```python
from build123d import *

# Parameters (mm, degrees)
SKETCH2_R               = 27.178
BOSS_EXTRUDE1_DEPTH     = 10
BOSS_EXTRUDE2_START     = -28
BOSS_EXTRUDE2_DEPTH     = 28
SHELL1_START            = -10
SHELL1_DEPTH            = 36
SHELL1_2_DEPTH          = 8
CUT_EXTRUDE3_DEPTH      = 10
CUT_EXTRUDE4_DEPTH      = 47.115916344
CUT_EXTRUDE4_DEPTH_BACK = 47.115916344
SKETCH6_R               = 1.75
SKETCH7_R               = 4
CUT_EXTRUDE6_DEPTH      = 47.115916478


# Read off the part's stored shape, not the designer's step: Shell1
with BuildPart() as part:
    # Sketch2 → Boss-Extrude1 (new body)
    with BuildSketch(Plane(origin=(0, 0, 0), x_dir=(1, 0, 0), z_dir=(0, 1, 0))):
        with Locations(Location((0, 0, 0), (0, 0, 270))):
            Circle(SKETCH2_R)
    extrude(amount=-BOSS_EXTRUDE1_DEPTH)

    # Sketch3 → Boss-Extrude2 (add)
    with BuildSketch(Plane(origin=(0, 0, 0), x_dir=(-1, 0, 0), z_dir=(0, -1, 0)).offset(BOSS_EXTRUDE2_START)):
        with BuildLine():
            Line((-23.587998728, 13.5), (-20.913788663, 13.5))
            ThreePointArc((-20.913788663, 13.5), (-13.609833087, 20.842480649), (-3.95, 24.57710431))
            Line((-3.95, 24.57710431), (-3.95, 20))
            ThreePointArc((-3.95, 20), (0, 16.05), (3.95, 20))
            Line((3.95, 20), (3.95, 24.57710431))
            ThreePointArc((3.95, 24.57710431), (13.609833087, 20.842480649), (20.913788663, 13.5))
            Line((20.913788663, 13.5), (23.587998728, 13.5))
            ThreePointArc((23.587998728, 13.5), (27.178, 0), (23.587998728, -13.5))
            Line((23.587998728, -13.5), (20.913788663, -13.5))
            ThreePointArc((20.913788663, -13.5), (13.609833087, -20.842480649), (3.95, -24.57710431))
            Line((3.95, -24.57710431), (3.95, -20))
            ThreePointArc((3.95, -20), (0, -16.05), (-3.95, -20))
            Line((-3.95, -20), (-3.95, -24.57710431))
            ThreePointArc((-3.95, -24.57710431), (-13.609833087, -20.842480649), (-20.913788663, -13.5))
            Line((-20.913788663, -13.5), (-23.587998728, -13.5))
            ThreePointArc((-23.587998728, -13.5), (-27.178, 0), (-23.587998728, 13.5))
        make_face()
    extrude(amount=BOSS_EXTRUDE2_DEPTH)

    # Shell1 outline → Shell1 (cut)
    with BuildSketch(Plane(origin=(0, 0, 0), x_dir=(1, 0, 0), z_dir=(0, 1, 0)).offset(SHELL1_START)):
        with BuildLine():
            ThreePointArc((22.398251807, -11.5), (25.178, 0), (22.398251807, 11.5))
            Line((22.398251807, 11.5), (19.794356677, 11.5))
            ThreePointArc((19.794356677, 11.5), (13.921689669, 18.172867496), (5.95, 22.105747132))
            Line((5.95, 22.105747132), (5.95, 20))
            ThreePointArc((5.95, 20), (0, 14.05), (-5.95, 20))
            Line((-5.95, 20), (-5.95, 22.105747132))
            ThreePointArc((-5.95, 22.105747132), (-13.921689669, 18.172867496), (-19.794356677, 11.5))
            Line((-19.794356677, 11.5), (-22.398251807, 11.5))
            ThreePointArc((-22.398251807, 11.5), (-25.178, 0), (-22.398251807, -11.5))
            Line((-22.398251807, -11.5), (-19.794356677, -11.5))
            ThreePointArc((-19.794356677, -11.5), (-13.921689669, -18.172867496), (-5.95, -22.105747132))
            Line((-5.95, -22.105747132), (-5.95, -20))
            ThreePointArc((-5.95, -20), (0, -14.05), (5.95, -20))
            Line((5.95, -20), (5.95, -22.105747132))
            ThreePointArc((5.95, -22.105747132), (13.921689669, -18.172867496), (19.794356677, -11.5))
            Line((19.794356677, -11.5), (22.398251807, -11.5))
        make_face()
    extrude(amount=SHELL1_DEPTH, mode=Mode.SUBTRACT)

    # Shell1 2 outline → Shell1 2 (cut)
    with BuildSketch(Plane(origin=(0, 0, 0), x_dir=(1, 0, 0), z_dir=(0, 1, 0)).offset(SHELL1_START)):
        with BuildLine():
            Line((19.794356677, 11.5), (22.398251807, 11.5))
            ThreePointArc((22.398251807, 11.5), (0, 25.178), (-22.398251807, 11.5))
            Line((-22.398251807, 11.5), (-19.794356677, 11.5))
            ThreePointArc((-19.794356677, 11.5), (-13.921689669, 18.172867496), (-5.95, 22.105747132))
            Line((-5.95, 22.105747132), (-5.95, 20))
            ThreePointArc((-5.95, 20), (0, 14.05), (5.95, 20))
            Line((5.95, 20), (5.95, 22.105747132))
            ThreePointArc((5.95, 22.105747132), (13.921689669, 18.172867496), (19.794356677, 11.5))
        make_face()
        with BuildLine():
            ThreePointArc((-22.398251807, -11.5), (0, -25.178), (22.398251807, -11.5))
            Line((22.398251807, -11.5), (19.794356677, -11.5))
            ThreePointArc((19.794356677, -11.5), (13.921689669, -18.172867496), (5.95, -22.105747132))
            Line((5.95, -22.105747132), (5.95, -20))
            ThreePointArc((5.95, -20), (0, -14.05), (-5.95, -20))
            Line((-5.95, -20), (-5.95, -22.105747132))
            ThreePointArc((-5.95, -22.105747132), (-13.921689669, -18.172867496), (-19.794356677, -11.5))
            Line((-19.794356677, -11.5), (-22.398251807, -11.5))
        make_face()
    extrude(amount=SHELL1_2_DEPTH, mode=Mode.SUBTRACT)

    # Sketch5 → Cut-Extrude3 (cut)
    with BuildSketch(Plane(origin=(0, -10, 0), x_dir=(1, 0, 0), z_dir=(0, 1, 0))):
        with BuildLine():
            Line((-23.587998728, 13.5), (-21.252804144, 13.5))
            ThreePointArc((-21.252804144, 13.5), (-21.848424918, 12.513113625), (-22.398251807, 11.5))
            Line((-22.398251807, 11.5), (22.398251807, 11.5))
            ThreePointArc((22.398251807, 11.5), (21.848424918, 12.513113625), (21.252804144, 13.5))
            Line((21.252804144, 13.5), (23.587998728, 13.5))
            ThreePointArc((23.587998728, 13.5), (0, 27.178), (-23.587998728, 13.5))
        make_face()
    cut_extrude3 = extrude(amount=CUT_EXTRUDE3_DEPTH, mode=Mode.SUBTRACT)

    # Mirror1: Cut-Extrude3 across plane
    add(cut_extrude3.mirror(Plane.XY), mode=Mode.SUBTRACT)

    # Sketch6 → Cut-Extrude4 (cut, two sides: drawn at the far end of the back side and taken through both)
    with BuildSketch(Plane(origin=(0, 0, 0), x_dir=(0, 0, -1), z_dir=(1, 0, 0)).offset(-CUT_EXTRUDE4_DEPTH_BACK)):
        with Locations((0, -5)):
            Circle(SKETCH6_R)
    extrude(amount=CUT_EXTRUDE4_DEPTH + CUT_EXTRUDE4_DEPTH_BACK, mode=Mode.SUBTRACT)

    # Sketch7 → Cut-Extrude6 (cut, through all)
    with BuildSketch(Plane(origin=(0, 0, 0), x_dir=(1, 0, 0), z_dir=(0, 1, 0))):
        with Locations(Location((0, 0, 0), (0, 0, 90))):
            Circle(SKETCH7_R)
    extrude(amount=CUT_EXTRUDE6_DEPTH, mode=Mode.SUBTRACT)


solid = part.part
```
The listing builds one solid part. Answer for the finished solid, in the listing's coordinates (mm). A direction names the side the tool comes from. Give positions to 0.01 mm unless a question says otherwise; leave off trailing zeros. Write each loop counter-clockwise with the first axis right and the second up, starting at its lowest first coordinate (ties: lowest second). Pieces come first, ordered by that corner, then holes. Notation, with made-up numbers: (50.5, 61) - (93.5, 61) arc R17 ccw to (93.5, 87) - close; hole circle Ø6 at (82, 41). An arc over 180 degrees is marked (long way). Use one line per item in the form item = value. Start each with the question number.
1) Find section A-A on z = 0. Determine the outline of the cut face in (x, y).
2) Find section C-C on z = 19. Determine the outline of the cut face in (x, y).
3) Consider line 1 along X through (y, z) = (21, 16); line 2 along X through (y, z) = (27.1, 0); line 3 along Y through (x, z) = (25.7, 0). Determine where each line is inside the solid, lowest interval first. Write a range as from..to.
4) Flat-ended cylindrical pins translate along their axes: pin 1 Ø1.3 at (x, y) = (-21.5, 18.5) entering from -Z; pin 2 Ø6 at (x, z) = (4, 8) entering from -Y; pin 3 Ø10.5 at (x, z) = (-3, 20.5) entering from -Y. Find the tip coordinate at first contact, or state that the pin passes through.
5) A tool of negligible diameter and unlimited length cuts with its end or side. For faces 4 (the face through (-21, 13, -11.5)), 5 (the face through (22, 9, 13.5)), 6 (the face through (3.95, 14, -22)), from which of +Z, -Z, +X, -X, +Y, -Y can it reach the whole face along a straight path? Write none if from no direction.
6) The mould has two halves that part along Y. Classify faces 1 (the face through (26, -10, 0)), 2 (the face through (26.13, -6.71, 0.38)), 3 (the face through (-0.13, 12.82, 14.05)): pulls with the +Y half, pulls with the -Y half, needs draft (parallel to the pull), parting line crosses it, or undercut.
7) Find section B-B on y = -5. Determine the outline of the cut face in (x, z), plus the area to 3 significant figures.
8) Find section D-D on x = -14. Determine the outline of the cut face in (y, z).
Geometry results:
q1.outline = (-27.18, -10) - (-25.18, -10) - (-25.18, -6.75) - (-27.18, -6.75) - close; (-27.18, -3.25) - (-25.18, -3.25) - (-25.18, 26) - (-4, 26) - (-4, 28) - (-27.18, 28) - close; (4, 26) - (25.18, 26) - (25.18, -3.25) - (27.18, -3.25) - (27.18, 28) - (4, 28) - close; (25.18, -10) - (27.18, -10) - (27.18, -6.75) - (25.18, -6.75) - close
q2.outline = (-16.08, 0) - (-12.77, 0) - (-12.77, 26) - (-5.87, 26) - (-5.87, 0) - (-3.82, 0) - (-3.82, 28) - (-16.08, 28) - close; (3.82, 0) - (5.87, 0) - (5.87, 26) - (12.77, 26) - (12.77, 0) - (16.08, 0) - (16.08, 28) - (3.82, 28) - close
q3.line_1 = -19.07..-16.37, -4.4..4.4, 16.37..19.07
q3.line_2 = -27.18..-4, 4..27.18
q3.line_3 = -10..-6.75, -3.25..28
q4.pin_1 = -13.6
q4.pin_2 = 26
q4.pin_3 = 0
q5.face_4 = -Y
q5.face_5 = +Z, +X, +Y, -Y
q5.face_6 = -Z, +Y, -Y
q6.face_1 = pulls with the -Y half
q6.face_2 = undercut
q6.face_3 = needs draft
q7.outline = (-27.12, -1.75) arc R27.18 ccw to (-23.59, -13.5) - (-21.25, -13.5) arc R25.18 cw to (-25.12, -1.75) - close; (-27.12, 1.75) - (-25.12, 1.75) arc R25.18 cw to (-21.25, 13.5) - (-23.59, 13.5) arc R27.18 ccw to start; (21.25, -13.5) - (23.59, -13.5) arc R27.18 ccw to (27.12, -1.75) - (25.12, -1.75) arc R25.18 cw to start; (21.25, 13.5) arc R25.18 cw to (25.12, 1.75) - (27.12, 1.75) arc R27.18 ccw to (23.59, 13.5) - close
q7.area = 99.5 mm2
q8.outline = (0, -20.58) - (28, -20.58) - (28, 20.58) - (0, 20.58) - (0, 18.11) - (26, 18.11) - (26, -18.11) - (0, -18.11) - close
